For this review, use the dimensioned drawing (mm, ordinates from the lowest corner) and the shaded views. A direction names the side the tool comes from. Coordinates: 2 decimals unless noted, no trailing zeros. Loops run counter-clockwise (first coordinate to the right, second up) from the corner with the lowest first, then second, coordinate; pieces in that order, holes last. Notation, with made-up numbers: M 55,-14 L 66,-14 A25 ccw 66,12 Z; hole C 67.5,31.5 d5. An arc over 180 degrees is marked long. One line per item, written item: value.
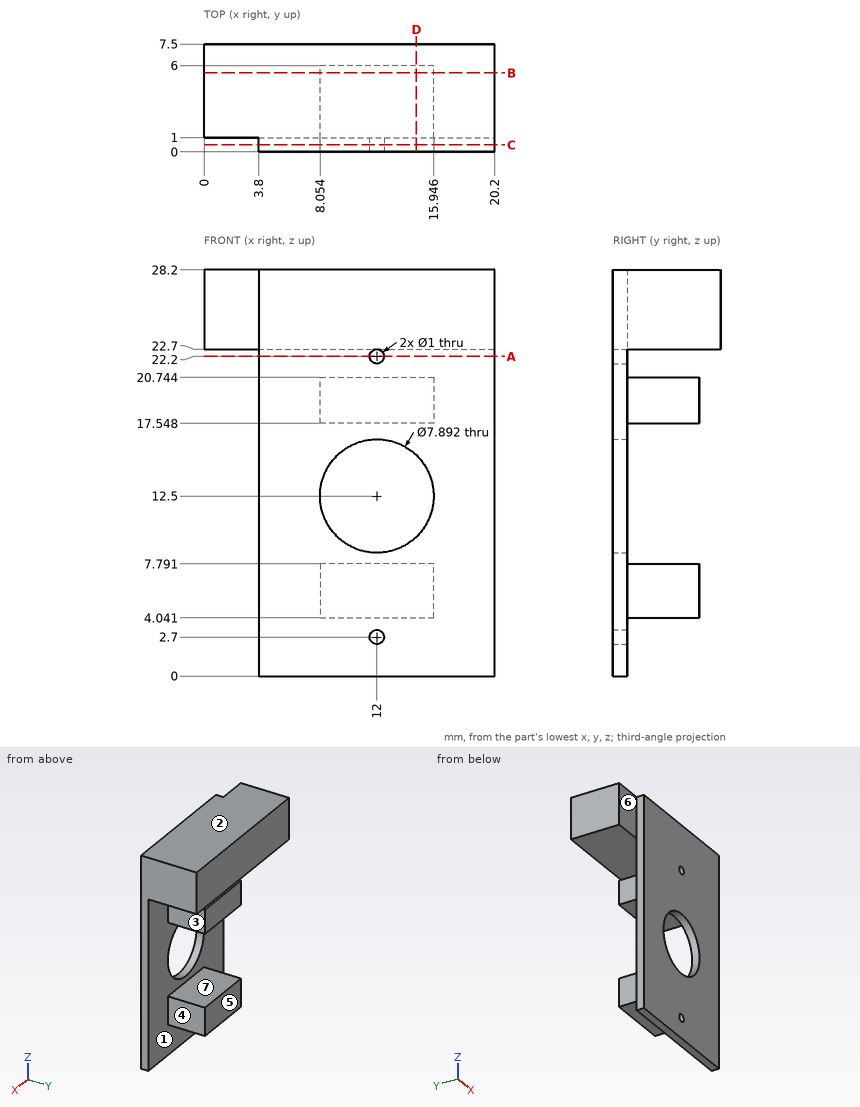
(1) To check wall thickness, follow L1, parallel to Z at x = 9.5, y = 5.25; L2, parallel to Z at x = 12, y = 0.3; L3, parallel to X at y = 0.4, z = 2.7. State the ranges of each line that lie inside material, in increasing order. Write a range as [from, to].
Checks:
L1: [4.04, 7.79], [17.55, 20.74], [22.7, 28.2]
L2: [0, 2.2], [3.2, 8.55], [16.45, 21.7], [22.7, 28.2]
L3: [3.8, 11.5], [12.5, 20.2]
(2) Insertion check: pin 1 Ø1.6 at (x, z) = (13, 19.5) entering from +Y; pin 2 Ø1.9 at (y, z) = (2.5, 6) entering from +X; pin 3 Ø1.1 at (y, z) = (0.5, 21) entering from -X. Each pin has a flat end and moves straight along its axis. Give the tip position at first contact, or say it passes through.
Checks:
pin 1: y = 6
pin 2: x = 15.95
pin 3: x = 3.8
(3) Draft analysis for pull direction Z (two halves, no side actions). For the marked faces 1, 2 and 3, state which applies: pulls with the +Z half, pulls with the -Z half, needs draft (parallel to the pull), parting line crosses it, or undercut.
Checks:
face 1: undercut
face 2: pulls with the +Z half
face 3: needs draft
(4) Add section C-C on y = 0.5. State the section outline as (x, z) points, then the cut area to 3 significant figures.
Checks:
outline: M 3.8,0 L 20.2,0 L 20.2,28.2 L 3.8,28.2 Z; hole C 12,12.5 d7.89; hole C 12,2.7 d1; hole C 12,22.2 d1
area: 412 mm^2
(5) Tool access review of the marked faces 4, 5, 6 and 7: name each direction out of +Z, -Z, +X, -X, +Y, -Y from which nothing blocks a thin tool from reaching the whole face with its end or side.
Checks:
face 4: -Z, +X, +Y
face 5: -Z, +X, -X, +Y
face 6: +Z, -Z, -X, -Y
face 7: +X, -X, +Y
(6) Add section D-D on x = 14.75. State the section outline as (y, z) points.
Checks:
outline: M 0,0 L 1,0 L 1,4.04 L 6,4.04 L 6,7.79 L 1,7.79 L 1,9.67 L 0,9.67 Z; M 0,15.33 L 1,15.33 L 1,17.55 L 6,17.55 L 6,20.74 L 1,20.74 L 1,22.7 L 7.5,22.7 L 7.5,28.2 L 0,28.2 Z
(7) Add section B-B on y = 5.5. State the section outline as (x, z) points, then the cut area to 3 significant figures.
Checks:
outline: M 0,22.7 L 20.2,22.7 L 20.2,28.2 L 0,28.2 Z; M 8.05,4.04 L 15.95,4.04 L 15.95,7.79 L 8.05,7.79 Z; M 8.05,17.55 L 15.95,17.55 L 15.95,20.74 L 8.05,20.74 Z
area: 166 mm^2
(8) Add section A-A on z = 22.2. State the section outline as (x, y) points.
Checks:
outline: M 3.8,0 L 11.5,0 L 11.5,1 L 3.8,1 Z; M 12.5,0 L 20.2,0 L 20.2,1 L 12.5,1 Z
